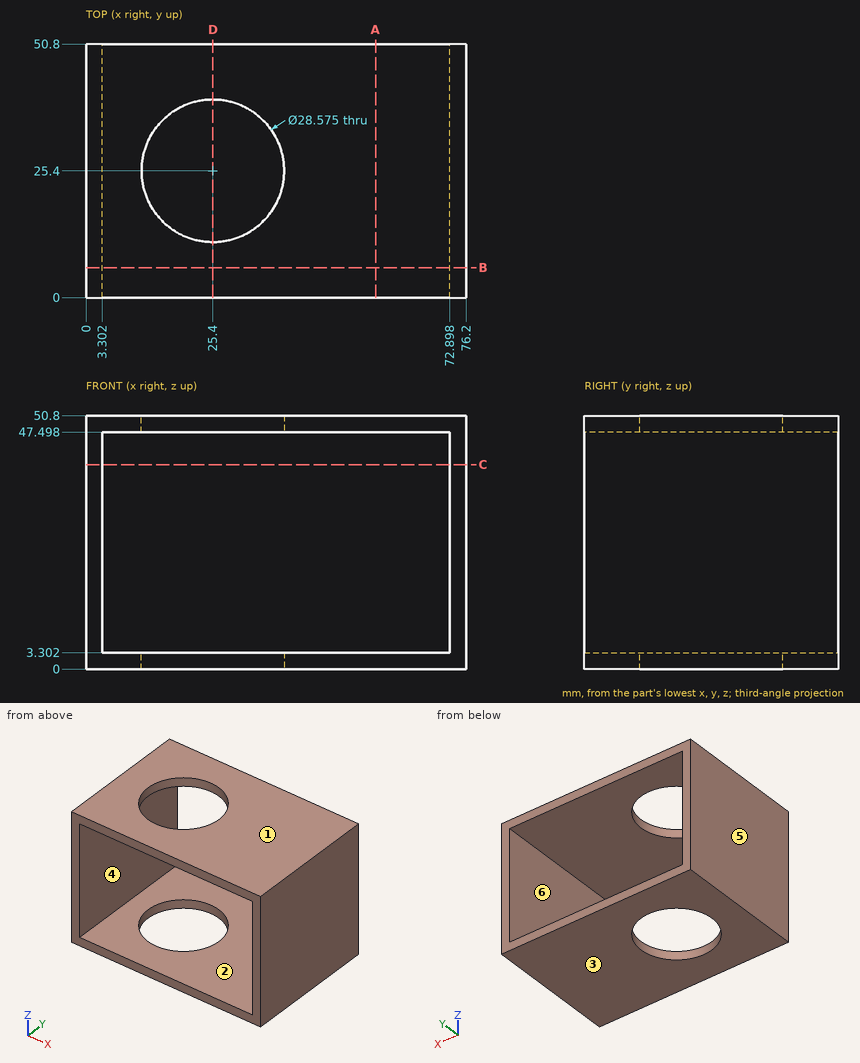
Check sheet for the drawn part. Datum: minimum x, y, z corner. Units: mm. A direction names the side the tool comes from. Coordinates: 2 decimals unless noted, no trailing zeros. Order: outer loops, then holes, each group sorted by start corner. A loop starts at its lowest first (then second) coordinate and runs counter-clockwise, first axis right, second up. Notation, with made-up numbers: M 49,-34.75 L 64,-34.75 A32 ccw 64,0.25 Z; hole C 59,-2 d7. An arc over 180 degrees is marked long. One line per item, written item: value. Start each with the question number.
Item 1: Access from +Z, -Z, +X, -X, +Y, -Y to the whole of each face (thin tool, end or side, straight path). Record for the marked faces 1 and 2.
Item 2: Mould release check, pull along X, two halves, no side actions. Record for the marked faces 3, 4, 5 and 6: released by +X, released by -X, zero draft, split by the parting line, or undercut.
Item 3: Scan lines: probe 1 along X at (y, z) = (25.4, 50.1); probe 2 along Z at (x, y) = (48.5, 4); probe 3 along X at (y, z) = (43, 4). Record each from-to range of solid material in increasing order.
Item 4: Sectioned sample at C-C (z = 41). Enter the section's corners in (x, y).
Item 5: Sectioned sample at D-D (x = 25.4). Enter the section's corners in (y, z).
Item 6: Sectioned sample at B-B (y = 6). Enter the section's corners in (x, z), then the cut area to 3 significant figures.
Item 7: Sectioned sample at A-A (x = 58). Enter the section's corners in (y, z), then the cut area to 3 significant figures.
Conclusion:
1. face 1: +Z, +X, -X, +Y, -Y
1. face 2: +Y, -Y
2. face 3: zero draft
2. face 4: undercut
2. face 5: released by -X
2. face 6: undercut
3. probe 1: x = 0 to 11.11, 39.69 to 76.2
3. probe 2: z = 0 to 3.3, 47.5 to 50.8
3. probe 3: x = 0 to 3.3, 72.9 to 76.2
4. outline: M 0,0 L 3.3,0 L 3.3,50.8 L 0,50.8 Z; M 72.9,0 L 76.2,0 L 76.2,50.8 L 72.9,50.8 Z
5. outline: M 0,0 L 11.11,0 L 11.11,3.3 L 0,3.3 Z; M 0,47.5 L 11.11,47.5 L 11.11,50.8 L 0,50.8 Z; M 39.69,0 L 50.8,0 L 50.8,3.3 L 39.69,3.3 Z; M 39.69,47.5 L 50.8,47.5 L 50.8,50.8 L 39.69,50.8 Z
6. outline: M 0,0 L 76.2,0 L 76.2,50.8 L 0,50.8 Z; hole M 3.3,3.3 L 72.9,3.3 L 72.9,47.5 L 3.3,47.5 Z
6. area: 795 mm^2
7. outline: M 0,0 L 50.8,0 L 50.8,3.3 L 0,3.3 Z; M 0,47.5 L 50.8,47.5 L 50.8,50.8 L 0,50.8 Z
7. area: 335 mm^2
